Can you work these out from the model? Positions are in its coordinate system, mm. Give positions to 0.01 mm unless a question says otherwise; leave off trailing zeros. Order: outer loops, then holes, each group sorted by start corner. A loop starts at its lowest first (then second) coordinate and runs counter-clockwise, first axis right, second up. Notation, with made-up numbers: M 82,0 L 129,0 A22 ccw 129,34 Z; hole C -39.75,30.25 d9. An arc over 180 degrees is marked long. Answer as a JSON object with one key per item and string values.
```python
from build123d import *

# Parameters (mm, degrees)
SKETCH1_R             = 25
BOSS_EXTRUDE1_DEPTH   = 1.8
BOSS_EXTRUDE1_2_DEPTH = 1.8
BOSS_EXTRUDE1_3_DEPTH = 1.8
BOSS_EXTRUDE2_DEPTH   = 1.4


with BuildPart() as part:
    # Sketch1 → Boss-Extrude1 (new body)
    with BuildSketch(Plane(origin=(0, 0, 0), x_dir=(1, 0, 0), z_dir=(0, 1, 0))):
        with BuildLine():
            ThreePointArc((1, 18.018524874), (0, 72), (-1, 18.018524874))
            ThreePointArc((-1, 18.018524874), (0, 18), (1, 18.018524874))
        make_face()
        with Locations(Location((0, 45, 0), (0, 0, 270))):
            Circle(SKETCH1_R, mode=Mode.SUBTRACT)
    extrude(amount=BOSS_EXTRUDE1_DEPTH)



with BuildPart() as body_2:
    # Sketch1 → Boss-Extrude1 2 (new body)
    with BuildSketch(Plane(origin=(0, 0, 0), x_dir=(1, 0, 0), z_dir=(0, 1, 0))):
        with BuildLine():
            ThreePointArc((18.018524874, 1), (72, 0), (18.018524874, -1))
            ThreePointArc((18.018524874, -1), (18, 0), (18.018524874, 1))
        make_face()
        with Locations(Location((45, 0, 0), (0, 0, 270))):
            Circle(SKETCH1_R, mode=Mode.SUBTRACT)
    extrude(amount=BOSS_EXTRUDE1_2_DEPTH)


with BuildPart() as body_3:
    # Sketch1 → Boss-Extrude1 3 (new body)
    with BuildSketch(Plane(origin=(0, 0, 0), x_dir=(1, 0, 0), z_dir=(0, 1, 0))):
        with BuildLine():
            ThreePointArc((-1, 3.872983346), (0, 4), (1, 3.872983346))
            ThreePointArc((1, 3.872983346), (2.828427125, 2.828427125), (3.872983346, 1))
            ThreePointArc((3.872983346, 1), (4, 0), (3.872983346, -1))
            ThreePointArc((3.872983346, -1), (3.473184708, -1.984184464), (2.828427125, -2.828427125))
            Line((2.828427125, -2.828427125), (-2.828427125, 2.828427125))
            ThreePointArc((-2.828427125, 2.828427125), (-1.984184464, 3.473184708), (-1, 3.872983346))
        make_face()
    extrude(amount=BOSS_EXTRUDE1_3_DEPTH)


with BuildPart() as part_1:
    add(part.part)

    add(body_2.part)  # Boss-Extrude2 merges body 2

    add(body_3.part)  # Boss-Extrude2 merges body 3
    # Sketch1_3 → Boss-Extrude2 (add)
    with BuildSketch(Plane(origin=(0, 0, 0), x_dir=(1, 0, 0), z_dir=(0, 1, 0))):
        with BuildLine():
            Line((-1, 18.018524874), (-1, 3.872983346))
            ThreePointArc((-1, 3.872983346), (0, 4), (1, 3.872983346))
            Line((1, 3.872983346), (1, 18.018524874))
            ThreePointArc((1, 18.018524874), (0, 18), (-1, 18.018524874))
        make_face()
        with BuildLine():
            ThreePointArc((18.018524874, 1), (18, 0), (18.018524874, -1))
            Line((18.018524874, -1), (3.872983346, -1))
            ThreePointArc((3.872983346, -1), (4, 0), (3.872983346, 1))
            Line((3.872983346, 1), (18.018524874, 1))
        make_face()
    extrude(amount=BOSS_EXTRUDE2_DEPTH)


solid = part_1.part
```
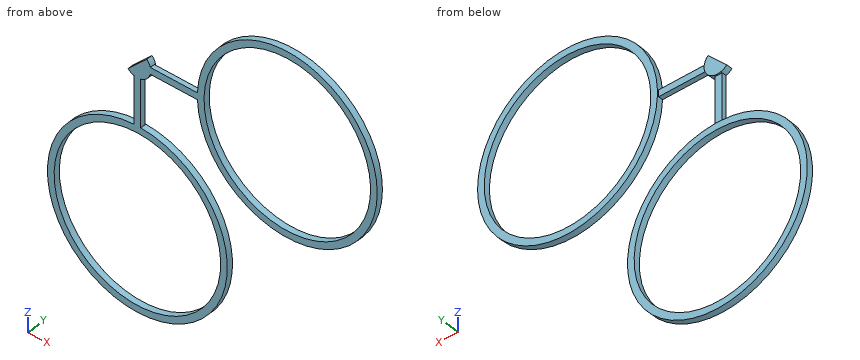
1) I want a section at B-B on y = 0.9. Write out the boundary of the cut face in (x, z), and give its area (3 significant figures).
Results found:
{"outline": "M -2.83,-2.83 A4 ccw -1,-3.87 L -1,-18.02 A27 ccw long 1,-18.02 L 1,-3.87 A4 ccw 3.87,-1 L 18.02,-1 A27 ccw long 18.02,1 L 3.87,1 A4 ccw 2.83,2.83 Z; hole C 0,-45 d50; hole C 45,0 d50", "area": "735 mm²"}
2) I want a section at D-D on x = 13. Write out the boundary of the cut face in (y, z), and give its area (3 significant figures).
Results found:
{"outline": "M 0,-68.66 L 1.8,-68.66 L 1.8,-66.35 L 0,-66.35 Z; M 0,-23.65 L 1.8,-23.65 L 1.8,-21.34 L 0,-21.34 Z; M 0,-1 L 1.4,-1 L 1.4,1 L 0,1 Z", "area": "11.1 mm²"}
3) I want a section at A-A on x = 45. Write out the boundary of the cut face in (y, z).
Results found:
{"outline": "M 0,-27 L 1.8,-27 L 1.8,-25 L 0,-25 Z; M 0,25 L 1.8,25 L 1.8,27 L 0,27 Z"}
4) I'm going to push flat-ended pins straight in: pin 1 Ø0.7 at (x, y) = (14, 0.5) entering from -Z; pin 2 Ø0.7 at (y, z) = (1, -8) entering from +X; pin 3 Ø1 at (x, z) = (0, -11) entering from +Y. Where does each tip first touch, or does it pass through?
Results found:
{"pin 1": "stops at z = -68.3", "pin 2": "stops at x = 70.89", "pin 3": "stops at y = 1.4"}
5) I need wall thicknesses on L1, parallel to X at y = 1.35, z = -45; L2, parallel to X at y = 1, z = 0; L3, parallel to Z at x = -13, y = 1.4. Which ranges of each line are inside material? Lowest first, please.
Results found:
{"L1": "x = -27 to -25, 25 to 27", "L2": "x = 0 to 20, 70 to 72", "L3": "z = -68.66 to -66.35, -23.65 to -21.34"}
6) I want a section at C-C on z = -45. Write out the boundary of the cut face in (x, y), and give its area (3 significant figures).
Results found:
{"outline": "M -27,0 L -25,0 L -25,1.8 L -27,1.8 Z; M 25,0 L 27,0 L 27,1.8 L 25,1.8 Z", "area": "7.20 mm²"}
